```python
from build123d import *

# Parameters (mm, degrees)
SKETCH1_W                     = 38.1
SKETCH1_H                     = 30.48
SKETCH1_R                     = 7.62
SKETCH1_R_2                   = 2.54
BOSS_EXTRUDE1_DEPTH           = 1.27
BOSS_EXTRUDE2_DEPTH           = 1.524
BOSS_EXTRUDE3_DEPTH           = 0.762
BOSS_EXTRUDE3_DRAFT           = -45
BOSS_EXTRUDE3_PROFILE_2_DEPTH = 0.762
BOSS_EXTRUDE3_PROFILE_2_DRAFT = -45
BOSS_EXTRUDE3_PROFILE_3_DEPTH = 0.762
BOSS_EXTRUDE3_PROFILE_3_DRAFT = -45
SKETCH6_W                     = 5.08
SKETCH6_H                     = 1.016
BOSS_EXTRUDE4_DEPTH           = 0.254


with BuildPart() as part:
    # Sketch1 → Boss-Extrude1 (new body)
    with BuildSketch(Plane(origin=(0, 0, 0), x_dir=(1, 0, 0), z_dir=(0, 1, 0))):
        Rectangle(SKETCH1_W, SKETCH1_H)
        with Locations(Location((0, 0, 0), (0, 0, 270))):
            Circle(SKETCH1_R, mode=Mode.SUBTRACT)
        with Locations(Location((12.7, -10.16, 0), (0, 0, 270))):
            Circle(SKETCH1_R_2, mode=Mode.SUBTRACT)
        with Locations(Location((-12.7, -10.16, 0), (0, 0, 270))):
            Circle(SKETCH1_R_2, mode=Mode.SUBTRACT)
    extrude(amount=BOSS_EXTRUDE1_DEPTH)

    # Sketch2 → Boss-Extrude2 (add)
    with BuildSketch(Plane(origin=(0, 0, 0), x_dir=(-1, 0, 0), z_dir=(0, -1, 0))):
        with BuildLine():
            ThreePointArc((-9.731051279, 2.921), (-10.16, 0), (-9.731051279, -2.921))
            Line((-9.731051279, -2.921), (-12.271051279, -2.921))
            Line((-12.271051279, -2.921), (-12.271051279, 2.921))
            Line((-12.271051279, 2.921), (-9.731051279, 2.921))
        make_face()
        with BuildLine():
            ThreePointArc((-3.81, -9.418572079), (0, -10.16), (3.81, -9.418572079))
            Line((3.81, -9.418572079), (3.81, -11.958572079))
            Line((3.81, -11.958572079), (-3.81, -11.958572079))
            Line((-3.81, -11.958572079), (-3.81, -9.418572079))
        make_face()
        with BuildLine():
            ThreePointArc((9.731051279, -2.921), (10.16, 0), (9.731051279, 2.921))
            Line((9.731051279, 2.921), (12.271051279, 2.921))
            Line((12.271051279, 2.921), (12.271051279, -2.921))
            Line((12.271051279, -2.921), (9.731051279, -2.921))
        make_face()
    extrude(amount=BOSS_EXTRUDE2_DEPTH)


with BuildPart() as boss_extrude3_tool:
    # Sketch4 → Boss-Extrude3 (with draft: the straight prism first)
    with BuildSketch(Plane(origin=(0, -1.524, 0), x_dir=(-1, 0, 0), z_dir=(0, -1, 0))):
        with BuildLine():
            ThreePointArc((3.81, -9.418572079), (0, -10.16), (-3.81, -9.418572079))
            Line((-3.81, -9.418572079), (-3.81, -11.958572079))
            Line((-3.81, -11.958572079), (3.81, -11.958572079))
            Line((3.81, -11.958572079), (3.81, -9.418572079))
        make_face()
    extrude(amount=BOSS_EXTRUDE3_DEPTH)
    # Boss-Extrude3: the draft: its side faces are tilted about the plane it starts from
    boss_extrude3_sides = [boss_extrude3_tool.faces().sort_by_distance(p)[0] for p in [
        (3.81, -1.905, 10.688572079),
        (0, -1.905, 11.958572079),
        (-3.81, -1.905, 10.688572079),
        (0, -1.905, 10.16),
    ]]
    draft(boss_extrude3_sides, Plane(origin=(0, -1.524, 0), x_dir=(-1, 0, 0), z_dir=(0, -1, 0)), BOSS_EXTRUDE3_DRAFT)


with BuildPart() as part_1:
    add(part.part)

    # Boss-Extrude3: add boss_extrude3_tool
    add(boss_extrude3_tool.part)


with BuildPart() as boss_extrude3_profile_2_tool:
    # Sketch4 → Boss-Extrude3 profile 2 (with draft: the straight prism first)
    with BuildSketch(Plane(origin=(0, -1.524, 0), x_dir=(-1, 0, 0), z_dir=(0, -1, 0))):
        with BuildLine():
            Line((12.271051279, 2.921), (9.731051279, 2.921))
            ThreePointArc((9.731051279, 2.921), (10.16, 0), (9.731051279, -2.921))
            Line((9.731051279, -2.921), (12.271051279, -2.921))
            Line((12.271051279, -2.921), (12.271051279, 2.921))
        make_face()
    extrude(amount=BOSS_EXTRUDE3_PROFILE_2_DEPTH)
    # Boss-Extrude3 profile 2: the draft: its side faces are tilted about the plane it starts from
    boss_extrude3_profile_2_sides = [boss_extrude3_profile_2_tool.faces().sort_by_distance(p)[0] for p in [
        (-11.001051279, -1.905, -2.921),
        (-10.16, -1.905, 0),
        (-11.001051279, -1.905, 2.921),
        (-12.271051279, -1.905, 0),
    ]]
    draft(boss_extrude3_profile_2_sides, Plane(origin=(0, -1.524, 0), x_dir=(-1, 0, 0), z_dir=(0, -1, 0)), BOSS_EXTRUDE3_PROFILE_2_DRAFT)


with BuildPart() as part_2:
    add(part_1.part)

    # Boss-Extrude3 profile 2: add boss_extrude3_profile_2_tool
    add(boss_extrude3_profile_2_tool.part)


with BuildPart() as boss_extrude3_profile_3_tool:
    # Sketch4 → Boss-Extrude3 profile 3 (with draft: the straight prism first)
    with BuildSketch(Plane(origin=(0, -1.524, 0), x_dir=(-1, 0, 0), z_dir=(0, -1, 0))):
        with BuildLine():
            Line((-9.731051279, 2.921), (-12.271051279, 2.921))
            Line((-12.271051279, 2.921), (-12.271051279, -2.921))
            Line((-12.271051279, -2.921), (-9.731051279, -2.921))
            ThreePointArc((-9.731051279, -2.921), (-10.16, 0), (-9.731051279, 2.921))
        make_face()
    extrude(amount=BOSS_EXTRUDE3_PROFILE_3_DEPTH)
    # Boss-Extrude3 profile 3: the draft: its side faces are tilted about the plane it starts from
    boss_extrude3_profile_3_sides = [boss_extrude3_profile_3_tool.faces().sort_by_distance(p)[0] for p in [
        (11.001051279, -1.905, -2.921),
        (12.271051279, -1.905, 0),
        (11.001051279, -1.905, 2.921),
        (10.16, -1.905, 0),
    ]]
    draft(boss_extrude3_profile_3_sides, Plane(origin=(0, -1.524, 0), x_dir=(-1, 0, 0), z_dir=(0, -1, 0)), BOSS_EXTRUDE3_PROFILE_3_DRAFT)


with BuildPart() as part_3:
    add(part_2.part)

    # Boss-Extrude3 profile 3: add boss_extrude3_profile_3_tool
    add(boss_extrude3_profile_3_tool.part)

    # Sketch6 → Boss-Extrude4 (add)
    with BuildSketch(Plane(origin=(0, 0, 0), x_dir=(-1, 0, 0), z_dir=(0, -1, 0))):
        with Locations((0, -8.128)):
            Rectangle(SKETCH6_W, SKETCH6_H)
        with Locations((0, -9.652)):
            Rectangle(SKETCH6_W, SKETCH6_H)
    extrude(amount=BOSS_EXTRUDE4_DEPTH)


solid = part_3.part
```
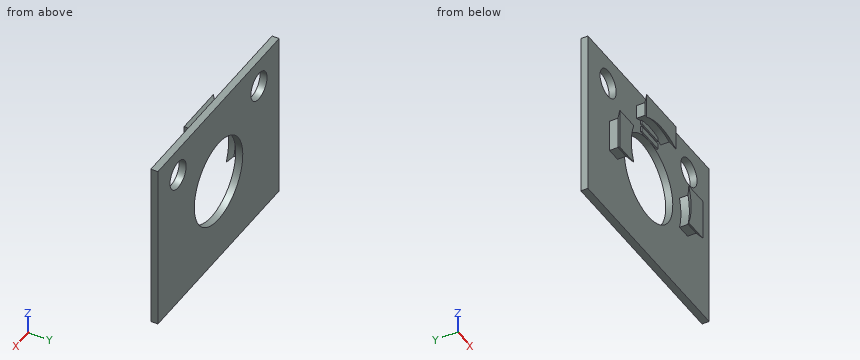
Can you work these out from the model? Positions are in its coordinate system, mm. Coordinates: 2 decimals unless noted, no trailing zeros. Loops run counter-clockwise (first coordinate to the right, second up) from the corner with the lowest first, then second, coordinate; pieces in that order, holes last.
1) For pin 1 (0.5 mm diameter, centred on y = -1, z = 0.5, fed in from -X); pin 2 (1.2 mm diameter, centred on x = -11.5, y = -1, fed in from -Z); pin 3 (0.8 mm diameter, centred on y = -0.5, z = 11, fed in from +X); pin 4 (2 mm diameter, centred on x = -2.5, y = -0.5, fed in from -Z), each with a flat end and sliding along its axis, tell me the tip position at first contact or that it passes through.
2) Imagine slicing it at C-C on z = 11.5. List the corners of the cut face in (x, y) for me.
3) Imagine slicing it at D-D on z = 5.5. List the corners of the cut face in (x, y) for me.
4) I need wall thicknesses on probe 1 along X at (y, z) = (0.9, 10.16); probe 2 along Y at (x, z) = (9, -2.5); probe 3 along X at (y, z) = (0.85, 3). Which ranges of each line are inside material? Lowest first, please.
5) Imagine slicing it at A-A on y = 0.5. List the corners of the cut face in (x, z) for me, plus the area to 3 significant figures.
6) Imagine slicing it at B-B on x = 5. List the corners of the cut face in (y, z) for me.
Completed:
1. pin 1: stops at x = -12.27
1. pin 2: stops at z = -3
1. pin 3: stops at x = 3.81
1. pin 4: stops at z = -15.24
2. outline: (-19.05, 0) - (-14.86, 0) - (-14.86, 1.27) - (-19.05, 1.27) - close; (-10.54, 0) - (-3.81, 0) - (-3.81, -1.52) - (-4.57, -2.29) - (4.57, -2.29) - (3.81, -1.52) - (3.81, 0) - (10.54, 0) - (10.54, 1.27) - (-10.54, 1.27) - close; (14.86, 0) - (19.05, 0) - (19.05, 1.27) - (14.86, 1.27) - close
3. outline: (-19.05, 0) - (-5.27, 0) - (-5.27, 1.27) - (-19.05, 1.27) - close; (5.27, 0) - (19.05, 0) - (19.05, 1.27) - (5.27, 1.27) - close
4. probe 1: x = -19.05 to -15.24, -10.16 to 10.16, 15.24 to 19.05
4. probe 2: y = 0 to 1.27
4. probe 3: x = -19.05 to -7, 7 to 19.05
5. outline: (-19.05, -15.24) - (19.05, -15.24) - (19.05, 15.24) - (-19.05, 15.24) - close; hole circle Ø5.08 at (-12.7, 10.16); hole circle Ø15.24 at (0, 0); hole circle Ø5.08 at (12.7, 10.16)
5. area: 938 mm2
6. outline: (0, -15.24) - (1.27, -15.24) - (1.27, -5.75) - (0, -5.75) - close; (0, 5.75) - (1.27, 5.75) - (1.27, 15.24) - (0, 15.24) - close
